Autodesk Inventor part; units mm, degrees
ref_plane "YZ Plane" through (0, 0, 0) normal (1, 0, 0) x (0, 1, 0)
ref_plane "XZ Plane" through (0, 0, 0) normal (0, 1, 0) x (-1, 0, 0)
ref_plane "XY Plane" through (0, 0, 0) normal (0, 0, 1) x (1, 0, 0)
sketch "Sketch1" plane through (0, 0, 0) normal (0, 1, 0) x (-1, 0, 0)
  line L0 (76.6044, 64.2788) -> (0, 0)
  line L1 (0, 0) -> (0, -40)
  dimension "d0" = 40
  dimension "d1" = 100
  dimension "d12" = 50
contour flange "Contour Flange1" sketch "Sketch1" thickness 3 bend radius 3 width 450 along (0, 1, 0) mid plane no both sides no wall seen from (-38.3022, 0, 32.1394) lies toward (0.6427876, 0, 0.7660444) curves L0 L1
bend "Bend1"
corner "Corner1"
sketch "Sketch2" plane through (-74.6761, 0, 66.5769) normal (0.6427876, 0, 0.7660444) x (0.7660444, 0, -0.6427876)
  line L0 (98.6011, 450) -> (98.6011, 0)
  line L1 (0, 450) -> (98.6011, 450)
  line L2 (0, 0) -> (0, 450)
  line L3 (0, 0) -> (98.6011, 0)
  line L4 (98.6011, 450) -> (0, 351.3989)
  line L5 (0, 98.6011) -> (98.6011, 0)
  dimension "d13" = 45
  dimension "d14" = 45
extrude "Extrusion1" cut sketch "Sketch2" against normal blind 10 contours L4 L2 L1 | L3 L2 L5
sketch "Sketch4" plane through (3, 0, -40) normal (1, 0, 0) x (0, 0, -1)
  line L0 (-38.6011, 450) -> (-38.6011, 0)
  line L1 (-38.6011, 450) -> (0, 450)
  line L2 (-19.3005, 112.5) -> (-19.3005, 225)
  line L3 (-19.3005, 225) -> (-19.3005, 337.5)
  point P0 (-40, 0)
  point P1 (-38.6011, 225)
  point P2 (-19.3005, 450)
  dimension "d17" = 112.5
hole "Hole1" at (3, 337.5, -20.6995) at (3, 225, -20.6995) at (3, 112.5, -20.6995) direction (-1, 0, 0) diameter 15 end through all
equation "\"d23\" = Thickness"
equation "\"d2\" = BendReliefWidth"
equation "\"d3\" = BendReliefDepth"
equation "\"d4\" = MinimumRemnant"
equation "\"d5\" = BendRadius"
equation "\"d7\" = BendRadius"
equation "\"d9\" = CornerReliefSize"
equation "\"d10\" = GapSize"
equation "\"d11\" = JacobiRadiusSize"
equation "\"BendRadius\" = Thickness"
equation "\"BendReliefWidth\" = Thickness"
equation "\"BendReliefDepth\" = 0.5 * Thickness"
equation "\"CornerReliefSize\" = 4 * Thickness"
equation "\"MinimumRemnant\" = 2 * Thickness"
equation "\"TransitionRadius\" = BendRadius"
equation "\"JacobiRadiusSize\" = BendRadius"
equation "\"GapSize\" = Thickness"
properties part number "SH3"
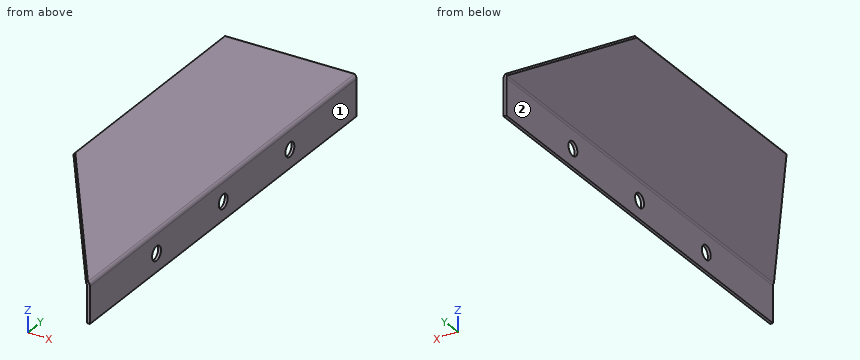
CAD build for the part. Positions are in the model's coordinates, mm. Face numbers are marked on the shaded views. A direction names the side the tool comes from. Round coordinates to 2 decimals unless told otherwise and drop trailing zeros. Write each loop counter-clockwise with the first axis right and the second up, starting at its lowest first coordinate (ties: lowest second). Pieces come first, ordered by that corner, then holes.
(1) Slice it at C-C, the plane y = 237.5. Write the cut outline in (x, z).
(2) Slice it at A-A, the plane y = 337.5. Write the cut outline in (x, z), and give its area (3 significant figures).
(3) 3-axis set-ups, long thin cutter, end or side, ignore diameter. For the marked faces 1 and 2: which of +Z, -Z, +X, -X, +Y, -Y reach the whole face in a straight line?
(4) Slice it at B-B, the plane z = -6.5. Write the cut outline in (x, y).
(5) Drop flat-ended pins along their axis: P1, Ø2, axis at x = -33, y = 213, coming from the -Z side; P2, Ø17, axis at y = 337.5, z = -20.7, coming from the -X side; P3, Ø1, axis at y = 286, z = 13, coming from the +X side. Give the stop position or say it passes through.
(6) Slice it at D-D, the plane x = -64. Write the cut outline in (y, z), and give its area (3 significant figures).
(7) Probe line 1 along Z through (x, y) = (0.85, 112.5); line 2 along Z through (x, y) = (0.75, 112.5); line 3 along X through (y, z) = (42.5, -20). List the from-to ranges inside material, lowest first.
From the geometry:
1. outline: (-76.6, 64.28) - (-1.07, 0.9) arc R3 cw to (0, -1.4) - (0, -40) - (3, -40) - (3, -1.4) arc R6 ccw to (0.86, 3.2) - (-74.68, 66.58) - close
2. outline: (-76.6, 64.28) - (-1.07, 0.9) arc R3 cw to (0, -1.4) - (0, -13.2) - (3, -13.2) - (3, -1.4) arc R6 ccw to (0.86, 3.2) - (-74.68, 66.58) - close; (0, -40) - (3, -40) - (3, -28.2) - (0, -28.2) - close
2. area: 378 mm2
3. face 1: +Z, -Z, +X, +Y, -Y
3. face 2: -Z, -X, +Y, -Y
4. outline: (0, 0) - (3, 0) - (3, 450) - (0, 450) - close
5. P1: stops at z = 26.85
5. P2: stops at x = 0
5. P3: stops at x = -10.23
6. outline: (82.15, 53.7) - (367.85, 53.7) - (365.34, 57.62) - (84.66, 57.62) - close
6. area: 1,110 mm2
7. line 1: z = -40 to -28.2, -13.2 to 3.2
7. line 2: z = -40 to -28.2, -13.2 to 3.29
7. line 3: x = 0 to 3
